```python
from build123d import *

# Parameters (mm, degrees)
SKETCH1_R                = 4
BOSS_EXTRUDE1_DEPTH      = 5
BOSS_EXTRUDE2_DEPTH      = 9
BOSS_EXTRUDE2_DEPTH_BACK = 9
SKETCH3_R                = 4
BOSS_EXTRUDE3_DEPTH      = 4.5
BOSS_EXTRUDE3_DEPTH_BACK = 4.5
SKETCH3_3_R              = 4


with BuildPart() as part:
    # Sketch1 → Boss-Extrude1 (new body)
    with BuildSketch(Plane.XY):
        with BuildLine():
            Line((-22, -15), (22, -15))
            ThreePointArc((22, -15), (27.656854249, -12.656854249), (30, -7))
            Line((30, -7), (30, 7))
            ThreePointArc((30, 7), (27.656854249, 12.656854249), (22, 15))
            Line((22, 15), (-22, 15))
            ThreePointArc((-22, 15), (-27.656854249, 12.656854249), (-30, 7))
            Line((-30, 7), (-30, -7))
            ThreePointArc((-30, -7), (-27.656854249, -12.656854249), (-22, -15))
        make_face()
        with Locations((-20, 0)):
            Circle(SKETCH1_R, mode=Mode.SUBTRACT)
        with Locations((20, 0)):
            Circle(SKETCH1_R, mode=Mode.SUBTRACT)
    extrude(amount=BOSS_EXTRUDE1_DEPTH)

    # Sketch3 → Boss-Extrude2 (add, two sides: drawn at the far end of the back side and taken through both)
    with BuildSketch(Plane(origin=(0, 0, 0), x_dir=(0, 0, -1), z_dir=(1, 0, 0)).offset(-BOSS_EXTRUDE2_DEPTH_BACK)):
        with BuildLine():
            ThreePointArc((-30.985266169, 4.608014794), (-31.839798327, 6.596210245), (-30.384833832, 8.198154275))
            Line((-30.384833832, 8.198154275), (-5, 15))
            Line((-5, 15), (-5, -15))
            Line((-5, -15), (-23.979362186, -15))
            ThreePointArc((-23.979362186, -15), (-25.637674581, -14.118033989), (-25.833411807, -12.25))
            ThreePointArc((-25.833411807, -12.25), (-25.423013471, -2.908363546), (-30.985266169, 4.608014794))
        make_face()
        with Locations((-38.81175916, -7)):
            Circle(SKETCH3_R)
    extrude(amount=BOSS_EXTRUDE2_DEPTH + BOSS_EXTRUDE2_DEPTH_BACK)


with BuildPart() as boss_extrude2_kept_piece:
    # of the separate pieces the step leaves, the one the design keeps (boss_extrude2_pieces_kept)
    add(part.part.solids().sort_by_distance((-22, -15, 0))[0])

    # Sketch3_3 → Boss-Extrude3 (add, two sides: drawn at the far end of the back side and taken through both)
    with BuildSketch(Plane(origin=(0, 0, 0), x_dir=(0, 0, -1), z_dir=(1, 0, 0)).offset(-BOSS_EXTRUDE3_DEPTH_BACK)):
        with BuildLine():
            Line((-30.384833832, 8.198154275), (-5, 15))
            Line((-5, 15), (-42.04675827, 5.074136854))
            ThreePointArc((-42.04675827, 5.074136854), (-50.885864002, -10.235118587), (-35.576521096, -19.074072829))
            Line((-35.576521096, -19.074072829), (-20.371874306, -15))
            Line((-20.371874306, -15), (-23.979362186, -15))
            ThreePointArc((-23.979362186, -15), (-25.637674581, -14.118033989), (-25.833411807, -12.25))
            ThreePointArc((-25.833411807, -12.25), (-25.423013471, -2.908363546), (-30.985266169, 4.608014794))
            ThreePointArc((-30.985266169, 4.608014794), (-31.839798327, 6.596210245), (-30.384833832, 8.198154275))
        make_face()
        with Locations((-38.81175916, -7)):
            Circle(SKETCH3_3_R, mode=Mode.SUBTRACT)
    extrude(amount=BOSS_EXTRUDE3_DEPTH + BOSS_EXTRUDE3_DEPTH_BACK)


solid = boss_extrude2_kept_piece.part
```
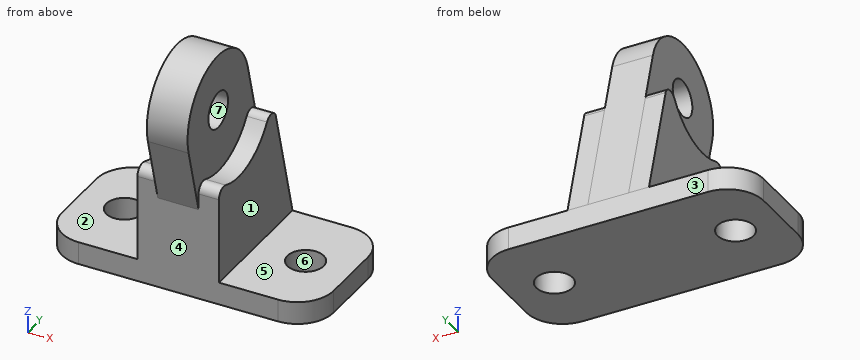
Geometry check sheet. Reference: the model listing, model coordinates, mm. Face numbers are marked on the shaded views. A direction names the side the tool comes from. Coordinates: 2 decimals unless noted, no trailing zeros. Order: outer loops, then holes, each group sorted by start corner. A loop starts at its lowest first (then second) coordinate and runs counter-clockwise, first axis right, second up. Notation, with made-up numbers: M 10,-29.75 L 42,-29.75 A35 cw 42,3.25 Z; hole C 2,27 d11. An arc over 180 degrees is marked long. Answer as a JSON object with one key per item and string values.
Q1. Cross-section at C-C on z = 41. Record the cut outline in (x, y), and give its area (3 significant figures).
Results are:
{"outline": "M -4.5,-19.31 L 4.5,-19.31 L 4.5,-10.35 L -4.5,-10.35 Z; M -4.5,-3.65 L 4.5,-3.65 L 4.5,5.35 L -4.5,5.35 Z", "area": "162 mm²"}
Q2. Scan lines: line 1 (Y direction, x = 20, z = 1.75); line 2 (Z direction, x = -19, y = -4); line 3 (X direction, y = 8.5, z = 7). Record each from-to range of solid material in increasing order.
Results are:
{"line 1": "y = -15 to -4, 4 to 15", "line 2": "z = 0 to 5", "line 3": "x = -9 to 9"}
Q3. Release check for a two-part mould opening along Y. For the marked faces 4, 5, 6 and 7 record: released by +Y, released by -Y, zero draft, split by the parting line, or undercut.
Results are:
{"face 4": "released by -Y", "face 5": "zero draft", "face 6": "undercut", "face 7": "undercut"}
Q4. Depth check by flat-ended pin: pin 1 Ø7 at (x, y) = (-20, 0) entering from -Z; pin 2 Ø3 at (y, z) = (-13, 17.5) entering from -X; pin 3 Ø12 at (x, z) = (1.5, 9.5) entering from -Y; pin 4 Ø9 at (y, z) = (-7, 38.81) entering from -X. Enter the tip coordinate at first touch or a pass-through.
Results are:
{"pin 1": "passes through", "pin 2": "stops at x = -9", "pin 3": "stops at y = -15", "pin 4": "stops at x = -4.5"}
Q5. Tool access check on the marked faces 1, 2 and 3. Record the directions out of +Z, -Z, +X, -X, +Y, -Y that give a thin tool (end or side, any length) a straight path to the whole face; none if there is none.
Results are:
{"face 1": "+Z, +X, +Y, -Y", "face 2": "+Z, -X, +Y, -Y", "face 3": "+Z, -Z, +X, -X, +Y"}
Q6. Cross-section at A-A on x = 20. Record the cut outline in (y, z).
Results are:
{"outline": "M -15,0 L -4,0 L -4,5 L -15,5 Z; M 4,0 L 15,0 L 15,5 L 4,5 Z"}
Q7. Cross-section at B-B on y = 0. Record the cut outline in (x, z), and give its area (3 significant figures).
Results are:
{"outline": "M -30,0 L -24,0 L -24,5 L -30,5 Z; M -16,0 L 16,0 L 16,5 L 9,5 L 9,26.69 L 4.5,26.69 L 4.5,49.17 L -4.5,49.17 L -4.5,26.69 L -9,26.69 L -9,5 L -16,5 Z; M 24,0 L 30,0 L 30,5 L 24,5 Z", "area": "813 mm²"}
